Model file for the job. Use its own axes, mm. A direction names the side the tool comes from. Coordinates: 2 decimals unless noted, no trailing zeros. Order: outer loops, then holes, each group sorted by start corner. A loop starts at its lowest first (then second) coordinate and runs counter-clockwise, first axis right, second up. Notation, with made-up numbers: (-29.75, 64.5) -> (0.25, 64.5) arc R12 cw to (0.25, 72.5) -> close; hole circle Ø3 at (39, 74). An arc over 180 degrees is marked (long way). Return JSON: item names as keys, results as strings. Group by question number.
1) Cut at D-D (x = 2.5). Write the cut outline in (y, z).
2) Flat gauge pins, fed straight in: pin 1 (2.5 mm diameter, centred on x = -26.99, z = 0, fed in from +Y); pin 2 (4 mm diameter, centred on x = 0, z = 26.99, fed in from +Y); pin 3 (6 mm diameter, centred on x = -23.5, y = 26, fed in from -Z); pin 4 (5 mm diameter, centred on y = 17, z = -17.5, fed in from +X). Where does each tip first touch, or does it go through?
3) Pull direction X, two halves, no side cores. Call faces 1 (the cylindrical face through (0.068, 52.535, -28.536)), 2 (the flat face through (0, -10, 0)): +X half, -X half, draft (parallel to the pull), parting line (faces both ways), or undercut.
4) Which spindle directions (+Z, -Z, +X, -X, +Y, -Y) get a long thin tool onto all of the face, cutting with end or side? Do faces 3 (the flat face through (0, 50, 27)), 4 (the flat face through (22, 55, -8)). Say none if no direction does.
5) Probe line 1 (X direction, y = -2.25, z = 0); line 2 (X direction, y = 20, z = 0) (3 decimals); line 3 (X direction, y = 47, z = 19). List the from-to ranges inside material, lowest first.
6) Cut at A-A (z = 0). State how many separate pieces and enclosed holes the cut face has, and give its area (3 significant figures).
7) Cut at C-C (y = 28.5). Write the cut outline in (x, z) (3 decimals).
8) Cut at B-B (x = -19.05). Write the cut outline in (y, z), and give its area (3 significant figures).
from build123d import *

# Parameters (mm, degrees)
SKETCH1_R           = 31.75
SKETCH1_R_2         = 22.225
BOSS_EXTRUDE1_DEPTH = 55
BOSS_EXTRUDE2_START = 10
SKETCH2_R           = 31.75
BOSS_EXTRUDE2_DEPTH = 10
SKETCH3_R           = 1.55
CUT_EXTRUDE1_DEPTH  = 5
SKETCH7_R           = 3
CUT_EXTRUDE2_DEPTH  = 10


with BuildPart() as part:
    # Sketch1 → Boss-Extrude1 (new body)
    with BuildSketch(Plane(origin=(0, 0, 0), x_dir=(1, 0, 0), z_dir=(0, 1, 0))):
        with Locations(Location((0, 0, 0), (0, 0, 270))):
            Circle(SKETCH1_R)
        with Locations(Location((0, 0, 0), (0, 0, 270))):
            Circle(SKETCH1_R_2, mode=Mode.SUBTRACT)
    extrude(amount=BOSS_EXTRUDE1_DEPTH)

    # Sketch2 → Boss-Extrude2 (add)
    with BuildSketch(Plane.XZ.offset(BOSS_EXTRUDE2_START)):
        with Locations(Location((0, 0, 0), (0, 0, 270))):
            Circle(SKETCH2_R)
    extrude(amount=-BOSS_EXTRUDE2_DEPTH)

    # Sketch3 → Cut-Extrude1 (cut)
    with BuildSketch(Plane(origin=(0, 55, 0), x_dir=(1, 0, 0), z_dir=(0, 1, 0))):
        with Locations(Location((0, 26.9875, 0), (0, 0, 270))):
            Circle(SKETCH3_R)
        with Locations(Location((26.9875, 0, 0), (0, 0, 270))):
            Circle(SKETCH3_R)
        with Locations(Location((0, -26.9875, 0), (0, 0, 270))):
            Circle(SKETCH3_R)
        with Locations(Location((-26.9875, 0, 0), (0, 0, 270))):
            Circle(SKETCH3_R)
    extrude(amount=-CUT_EXTRUDE1_DEPTH, mode=Mode.SUBTRACT)

    # Sketch7 → Cut-Extrude2 (cut)
    with BuildSketch(Plane(origin=(0, -10, 0), x_dir=(-1, 0, 0), z_dir=(0, -1, 0))):
        with Locations(Location((19.05, 0, 0), (0, 0, 90))):
            Circle(SKETCH7_R)
        with Locations(Location((-19.05, 0, 0), (0, 0, 90))):
            Circle(SKETCH7_R)
    extrude(amount=-CUT_EXTRUDE2_DEPTH, mode=Mode.SUBTRACT)


solid = part.part
Answers below:
{
 "1": {"outline": "(-10, -31.65) -> (55, -31.65) -> (55, -22.08) -> (0, -22.08) -> (0, 22.08) -> (55, 22.08) -> (55, 31.65) -> (-10, 31.65) -> close"},
 "2": {"pin 1": "stops at y = 50", "pin 2": "stops at y = 55", "pin 3": "stops at z = -24.24", "pin 4": "stops at x = 27.98"},
 "3": {"face 1": "undercut", "face 2": "draft"},
 "4": {"face 3": "+Y", "face 4": "+Z, -Z, +X, -X, +Y"},
 "5": {"line 1": "x = -31.75 to -22.05, -16.05 to 16.05, 22.05 to 31.75", "line 2": "x = -31.75 to -22.225, 22.225 to 31.75", "line 3": "x = -25.44 to -11.53, 11.53 to 25.44"},
 "6": {"separate pieces": "3", "enclosed holes": "0", "area": "1,530 mm^2"},
 "7": {"outline": "circle Ø63.5 at (0, 0); hole circle Ø44.45 at (0, 0)"},
 "8": {"outline": "(-10, -25.4) -> (55, -25.4) -> (55, -11.45) -> (0, -11.45) -> (0, -3) -> (-10, -3) -> close; (-10, 3) -> (0, 3) -> (0, 11.45) -> (55, 11.45) -> (55, 25.4) -> (-10, 25.4) -> close", "area": "1,980 mm^2"}
}
